Read the model definition and answer for the solid it produces. Units are mm, in the model's axes. Face numbers are marked on the shaded views. A direction names the side the tool comes from. Coordinates: 2 decimals unless noted, no trailing zeros. Order: outer loops, then holes, each group sorted by start corner. A loop starts at its lowest first (then second) coordinate and runs counter-clockwise, first axis right, second up. Notation, with made-up numbers: (23, 74.25) - (39, 74.25) arc R21 cw to (39, 108.25) - close; hole circle Ø8 at (70.5, 18). An arc over 180 degrees is marked (long way). Answer as a JSON object with one key per item and string values. Group by question number.
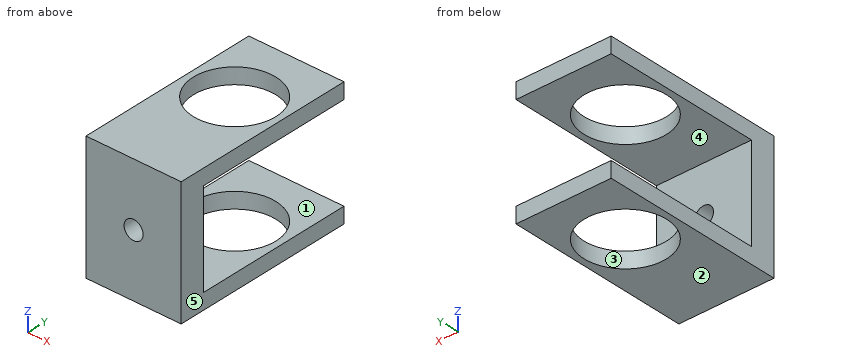
Autodesk Inventor part; units mm, degrees
ref_plane "YZ Plane" through (0, 0, 0) normal (1, 0, 0) x (0, 1, 0)
ref_plane "XZ Plane" through (0, 0, 0) normal (0, 1, 0) x (-1, 0, 0)
ref_plane "XY Plane" through (0, 0, 0) normal (0, 0, 1) x (1, 0, 0)
sketch "Sketch1" plane through (0, 0, 0) normal (0, 1, 0) x (-1, 0, 0)
  line L0 (-7.5, -10) -> (7.5, -10)
  line L1 (7.5, -10) -> (7.5, 10)
  line L2 (7.5, 10) -> (-7.5, 10)
  line L3 (-7.5, 10) -> (-7.5, -10)
  line L4 (-7.5, -10) -> (7.5, 10) construction
  line L5 (7.5, -10) -> (-7.5, 10) construction
  point P0 (0, 0)
  dimension "d0" = 15
  dimension "d1" = 20
extrude "Extrusion1" add sketch "Sketch1" along normal blind 4
sketch "Sketch2" plane through (0, 4, 0) normal (0, 1, 0) x (1, 0, 0)
  line L0 (-7.5, 10) -> (-7.5, -10)
  line L1 (7.5, -10) -> (7.5, 10)
  line L2 (-7.5, 10) -> (7.5, 10)
  line L3 (7.5, 10) -> (7.5, 7.5)
  line L4 (7.5, 7.5) -> (-7.5, 7.5)
  line L5 (-7.5, 7.5) -> (-7.5, 10)
  line L6 (7.5, 0) -> (0, 0) construction
  line L7 (-7.5, -10) -> (-7.5, 10)
  line L8 (7.5, 10) -> (7.5, -10)
  line L9 (-7.5, -10) -> (7.5, -10)
  line L10 (7.5, -7.5) -> (-7.5, -7.5)
  dimension "d4" = 2.5
extrude "Extrusion2" add sketch "Sketch2" along normal blind 25 contours L2 L1 L4 L0 | L10 L1 L9 L0
sketch "Sketch4" plane through (7.5, 0, -10) normal (0, 0, -1) x (-1, 0, 0)
  line L0 (7.5, 0) -> (7.5, 7) construction
  line L1 (0, 0) -> (0, 29) construction
  line L2 (15, 4) -> (15, 29) construction
  line L3 (0, 4) -> (0, 29) construction
  line L4 (15, 7) -> (0, 7) construction
  line L5 (0, 29) -> (15, 29) construction
  line L6 (15, 29) -> (0, 7) construction
  line L7 (0, 29) -> (15, 7) construction
  circle A0 centre (7.5, 18) radius 6.5
  dimension "d12" = 7
  dimension "d13" = 13
  dimension "d14" = 34.287
extrude "Extrusion4" cut sketch "Sketch4" against normal blind 25
sketch "Sketch5" plane through (0, 0, 0) normal (0, -1, 0) x (1, 0, 0)
  line L0 (-7.5, 10) -> (7.5, 10) construction
  line L1 (-7.5, 10) -> (7.5, -10) construction
  line L2 (7.5, 10) -> (-7.5, -10) construction
  circle A0 centre (0, 0) radius 1.5
  dimension "d17" = 3
extrude "Extrusion5" cut sketch "Sketch5" against normal blind 5
properties part number "llanta_1"
1. A cutting plane is placed at C-C on x = 0. Write down the section's boundary in (y, z).
2. For a pull along X with two mould halves and no side action, classify the marked faces 3, 4 and 5 as pulls with the +X half, pulls with the -X half, needs draft (parallel to the pull), parting line crosses it, or undercut.
3. Straight lines are drawn through the part: L1, parallel to Z at x = -4.25, y = 26.25; L2, parallel to Z at x = 0, y = 0.9; L3, parallel to Y at x = 4, z = 0. For each, find the intervals that lie inside material, in ascending order.
4. A cutting plane is placed at D-D on y = 18. Write down the section's boundary in (x, z).
5. A cutting plane is placed at B-B on x = -6. Write down the section's boundary in (y, z), and give its area (3 significant figures).
6. For the marked faces 1 and 2, determine the directions among +Z, -Z, +X, -X, +Y, -Y from which every point of the face is accessible in a straight line to the end or side of a thin tool.
7. Given pin 1 (1.5 mm diameter, centred on x = 3, z = -5, fed in from +Y); pin 2 (5 mm diameter, centred on y = 13, z = 4, fed in from +X), each flat-ended and moving along its own axis, determine where each tip first touches the part or whether it passes through.
8. A cutting plane is placed at A-A on y = 25. Write down the section's boundary in (x, z), and give its area (3 significant figures).
Derived:
{
 "1": {"outline": "(0, -10) - (11.5, -10) - (11.5, -7.5) - (4, -7.5) - (4, -1.5) - (0, -1.5) - close; (0, 1.5) - (4, 1.5) - (4, 7.5) - (11.5, 7.5) - (11.5, 10) - (0, 10) - close; (24.5, -10) - (29, -10) - (29, -7.5) - (24.5, -7.5) - close; (24.5, 7.5) - (29, 7.5) - (29, 10) - (24.5, 10) - close"},
 "2": {"face 3": "undercut", "face 4": "needs draft", "face 5": "pulls with the +X half"},
 "3": {"L1": "z = -10 to -7.5, 7.5 to 10", "L2": "z = -10 to -1.5, 1.5 to 10", "L3": "y = 0 to 4"},
 "4": {"outline": "(-7.5, -10) - (-6.5, -10) - (-6.5, -7.5) - (-7.5, -7.5) - close; (-7.5, 7.5) - (-6.5, 7.5) - (-6.5, 10) - (-7.5, 10) - close; (6.5, -10) - (7.5, -10) - (7.5, -7.5) - (6.5, -7.5) - close; (6.5, 7.5) - (7.5, 7.5) - (7.5, 10) - (6.5, 10) - close"},
 "5": {"outline": "(0, -10) - (15.5, -10) - (15.5, -7.5) - (4, -7.5) - (4, 7.5) - (15.5, 7.5) - (15.5, 10) - (0, 10) - close; (20.5, -10) - (29, -10) - (29, -7.5) - (20.5, -7.5) - close; (20.5, 7.5) - (29, 7.5) - (29, 10) - (20.5, 10) - close", "area": "180 mm2"},
 "6": {"face 1": "+X, -X, +Y", "face 2": "-Z, +X, -X, +Y, -Y"},
 "7": {"pin 1": "stops at y = 4", "pin 2": "passes through"},
 "8": {"outline": "(-7.5, -10) - (7.5, -10) - (7.5, -7.5) - (-7.5, -7.5) - close; (-7.5, 7.5) - (7.5, 7.5) - (7.5, 10) - (-7.5, 10) - close", "area": "75.0 mm2"}
}
